```python
from build123d import *

# Parameters (mm, degrees)
F1_DEPTH  = 31.52012
F0_R      = 3.9989944529
F0_R_2    = 4.0304935081
F2_DEPTH  = 10.8295
F3_DEPTH  = 11.66704
F0_R_3    = 9.2896599899
F4_DEPTH  = 31.97776
F6_R      = 7.7262681343
F6_R_2    = 5.87306791
F7_DEPTH  = 7.37838
F9_DEPTH  = 23.31858
F0_R_4    = 5.7595758306
F0_R_5    = 5.6310949549
F10_DEPTH = 19.41152
F0_W      = 10.16
F0_H      = 21.1746012493
F11_DEPTH = 19.65592


# Not quite as in the source:
# - a feature names something its author has since deleted; it is built from what else it names
# - the program builds the solid bodies; features that only make, move or delete a surface that nothing else refers to are left out


with BuildPart() as f1:
    # F0 (on Front) → F1 (new body)
    with BuildSketch(Plane.XZ):
        with BuildLine():
            Line((-32.945703147, 0), (-53.0377118984, 0))
            Line((-53.0377118984, 0), (-53.0377118984, -13.8332377828))
            Line((-53.0377118984, -13.8332377828), (-5.08, -13.8332377828))
            Line((-5.08, -13.8332377828), (5.08, -13.8332377828))
            Line((5.08, -13.8332377828), (53.0377118984, -13.8332377828))
            Line((53.0377118984, -13.8332377828), (53.0377118984, 0))
            Line((53.0377118984, 0), (32.945703147, 0))
            add(Edge.make_bspline(
                [(32.945703147, 0), (28.5647447129, 0.0625927983), (19.8735598839, 0.1867678132), (20.1720018391, 8.6992646442), (20.3200084018, 12.9208741543)],
                knots=[0, 0, 0, 0, 0.5040691828, 1, 1, 1, 1], degree=3))
            ThreePointArc((20.3200084018, 12.9208741543), (23.9781287511, 23.6330514006), (20.3200084018, 34.345228647))
            Line((20.3200084018, 34.345228647), (20.3200084018, 57.3156722881))
            Line((20.3200084018, 57.3156722881), (-18.3321793468, 57.3156722881))
            Line((-18.3321793468, 57.3156722881), (-18.3321793468, 34.345228647))
            ThreePointArc((-18.3321793468, 34.345228647), (-21.9102829622, 23.6330514006), (-18.3321793468, 12.9208741543))
            add(Edge.make_bspline(
                [(-32.945703147, 0), (-28.5122837396, 0.0592468916), (-19.728591274, 0.176629532), (-18.7947032642, 8.6996856696), (-18.3321793468, 12.9208741543)],
                knots=[0, 0, 0, 0, 0.5047329952, 1, 1, 1, 1], degree=3))
        make_face()
        with BuildLine():
            ThreePointArc((6.2648822412, 33.191720318), (12.6390408842, 27.6514544893), (15.0142637131, 19.5469643528))
            ThreePointArc((15.0142637131, 19.5469643528), (-7.6843579979, 6.6481753784), (-7.1484956716, 32.75026411))
            ThreePointArc((-7.1484956716, 32.75026411), (-0.4938765731, 34.5531031225), (6.2648822412, 33.191720318))
        make_face(mode=Mode.SUBTRACT)
    extrude(amount=F1_DEPTH)

    # F0 (on Front) → F2 (join)
    with BuildSketch(Plane.XZ):
        with BuildLine():
            Line((-18.3321793468, 62.8374100943), (-18.3321793468, 57.3156722881))
            Line((-18.3321793468, 57.3156722881), (20.3200084018, 57.3156722881))
            Line((20.3200084018, 57.3156722881), (20.3200084018, 62.8374100943))
            add(Edge.make_bspline(
                [(20.3200084018, 62.8374100943), (20.1052749574, 65.5197235908), (19.6543576651, 71.15229537), (13.2786405866, 71.4934853371), (9.9391337225, 71.6721956254)],
                knots=[0, 0, 0, 0, 0.4762147029, 1, 1, 1, 1], degree=3))
            Line((9.9391337225, 71.6721956254), (-5.7426103852, 71.6721956254))
            add(Edge.make_bspline(
                [(-18.3321793468, 62.8374100943), (-18.0134703448, 65.7269619482), (-17.326155356, 71.9584530192), (-9.7862501304, 71.772123737), (-5.7426103852, 71.6721956254)],
                knots=[0, 0, 0, 0, 0.4637015156, 1, 1, 1, 1], degree=3))
        make_face()
        with Locations((-10.6017430574, 65.7269619482)):
            Circle(F0_R, mode=Mode.SUBTRACT)
        with Locations((13.0313078181, 65.7087189627)):
            Circle(F0_R_2, mode=Mode.SUBTRACT)
    extrude(amount=F2_DEPTH)

    # F0 (on Front) → F3 (join)
    with BuildSketch(Plane.XZ):
        with BuildLine():
            Line((-18.3321793468, 34.345228647), (-53.0377118984, 0))
            Line((-53.0377118984, 0), (-32.945703147, 0))
            add(Edge.make_bspline(
                [(-32.945703147, 0), (-28.5122837396, 0.0592468916), (-19.728591274, 0.176629532), (-18.7947032642, 8.6996856696), (-18.3321793468, 12.9208741543)],
                knots=[0, 0, 0, 0, 0.5047329952, 1, 1, 1, 1], degree=3))
            ThreePointArc((-18.3321793468, 12.9208741543), (-21.9102829622, 23.6330514006), (-18.3321793468, 34.345228647))
        make_face()
        with BuildLine():
            Line((53.0377118984, 0), (20.3200084018, 34.345228647))
            ThreePointArc((20.3200084018, 34.345228647), (23.9781287511, 23.6330514006), (20.3200084018, 12.9208741543))
            add(Edge.make_bspline(
                [(32.945703147, 0), (28.5647447129, 0.0625927983), (19.8735598839, 0.1867678132), (20.1720018391, 8.6992646442), (20.3200084018, 12.9208741543)],
                knots=[0, 0, 0, 0, 0.5040691828, 1, 1, 1, 1], degree=3))
            Line((32.945703147, 0), (53.0377118984, 0))
        make_face()
    extrude(amount=F3_DEPTH)

    # F0 (on Front) → F4 (join)
    with BuildSketch(Plane.XZ):
        with BuildLine():
            ThreePointArc((-7.1484956716, 32.75026411), (-7.6843579979, 6.6481753784), (15.0142637131, 19.5469643528))
            ThreePointArc((15.0142637131, 19.5469643528), (12.6390408842, 27.6514544893), (6.2648822412, 33.191720318))
            ThreePointArc((6.2648822412, 33.191720318), (-0.4938765731, 34.5531031225), (-7.1484956716, 32.75026411))
        make_face()
        with Locations((0, 19.5469643528)):
            Circle(F0_R_3, mode=Mode.SUBTRACT)
    extrude(amount=F4_DEPTH)

    # F6 (on offset) → F7 (cut)
    with BuildSketch(Plane.XY.offset(50.8)):
        with Locations((0, -19.8897793889)):
            Circle(F6_R)
        with Locations((0, -19.8897793889)):
            Circle(F6_R_2, mode=Mode.SUBTRACT)
    extrude(amount=F7_DEPTH, mode=Mode.SUBTRACT)

    # F9 (cut): a face of the model
    f9_faces = [f1.faces().sort_by_distance(p)[0] for p in [
        (0, -19.8897793889, 57.3156722881),
    ]]
    extrude(f9_faces, amount=-F9_DEPTH, mode=Mode.SUBTRACT)

    # F0 (on Front) → F10 (join)
    with BuildSketch(Plane.XZ):
        with BuildLine():
            Line((-5.08, -13.8332377828), (-53.0377118984, -13.8332377828))
            Line((-53.0377118984, -13.8332377828), (-53.0377118984, -21.0930503504))
            add(Edge.make_bspline(
                [(-53.0377118984, -21.0930503504), (-53.4005944702, -25.2780429079), (-54.7251608325, -36.2581171884), (-35.7792689312, -35.346119388), (-25.8417483085, -35.0078390322)],
                knots=[0, 0, 0, 0, 0.3981682681, 1, 1, 1, 1], degree=3))
            Line((-25.8417483085, -35.0078390322), (-5.08, -35.0078390322))
            Line((-5.08, -35.0078390322), (-5.08, -13.8332377828))
        make_face()
        with Locations((-45.0574053683, -26.3939229293)):
            Circle(F0_R_4, mode=Mode.SUBTRACT)
        with BuildLine():
            Line((53.0377118984, -13.8332377828), (5.08, -13.8332377828))
            Line((5.08, -13.8332377828), (5.08, -35.0078390322))
            Line((5.08, -35.0078390322), (35.7808830812, -35.0078390322))
            add(Edge.make_bspline(
                [(53.0377118984, -21.0930503504), (52.1158724207, -25.6188280404), (49.8115979989, -34.1905224475), (41.3452471932, -34.893061815), (35.7808830812, -35.0078390322)],
                knots=[0, 0, 0, 0, 0.4907243677, 1, 1, 1, 1], degree=3))
            Line((53.0377118984, -21.0930503504), (53.0377118984, -13.8332377828))
        make_face()
        with Locations((43.7321887989, -26.8356617858)):
            Circle(F0_R_5, mode=Mode.SUBTRACT)
    extrude(amount=F10_DEPTH)

    # F0 (on Front) → F11 (join)
    with BuildSketch(Plane.XZ):
        with Locations((0, -24.4205384075)):
            Rectangle(F0_W, F0_H)
    extrude(amount=F11_DEPTH)


solid = f1.part
```
CAD build for the part. Positions are in the model's coordinates, mm. A direction names the side the tool comes from. Round coordinates to 2 decimals unless told otherwise and drop trailing zeros. Write each loop counter-clockwise with the first axis right and the second up, starting at its lowest first coordinate (ties: lowest second). Pieces come first, ordered by that corner, then holes.
Item 1: Band-saw the part on A-A on x = 0. Write the cut outline in (y, z), then the cut area to 3 significant figures.
Filled in:
outline: (-31.98, 4.53) - (-31.52, 4.53) - (-31.52, -13.83) - (-19.66, -13.83) - (-19.66, -35.01) - (0, -35.01) - (0, 10.26) - (-31.98, 10.26) - close; (-31.98, 28.84) - (0, 28.84) - (0, 71.67) - (-10.83, 71.67) - (-10.83, 57.32) - (-12.16, 57.32) - (-12.16, 50.8) - (-14.02, 50.8) - (-14.02, 34) - (-25.76, 34) - (-25.76, 50.8) - (-27.62, 50.8) - (-27.62, 57.32) - (-31.52, 57.32) - (-31.52, 34.56) - (-31.98, 34.56) - close
area: 1,940 mm2
Item 2: Mould opens along X. For faces 1 (the flat face through (20.32, -16, 45)), 2 (the flat face through (1, -10.83, 65)), 3 (the cylindrical face through (-0.765, -25.713, 42.516)) say: released by +X, released by -X, zero draft, split by the parting line, or undercut.
Filled in:
face 1: released by +X
face 2: zero draft
face 3: undercut
Item 3: Drill centre lines: L1, parallel to Z at x = 0, y = -21; L2, parallel to X at y = -2, z = 63.5; L3, parallel to Y at x = 24.5, z = -2.5. Where is each one in solid material? Low to high.
Filled in:
L1: z = -13.83 to 10.26, 28.84 to 34
L2: x = -18.26 to -13.92, -7.28 to 9.66, 16.4 to 20.27
L3: y = -31.52 to 0
Item 4: Band-saw the part on B-B on z = -10.5. Write the cut outline in (x, y).
Filled in:
outline: (-53.04, -31.52) - (53.04, -31.52) - (53.04, 0) - (-53.04, 0) - close
Item 5: Drop flat-ended pins along their axis: pin 1 Ø1 at (y, z) = (-5, 18) entering from -X; pin 2 Ø4 at (x, y) = (2, -23) entering from +Z; pin 3 Ø5 at (y, z) = (-25.5, 58) entering from -X; pin 4 Ø10 at (x, z) = (-23.5, 38.5) entering from -Y. Give the stop position or say it passes through.
Filled in:
pin 1: stops at x = -35.35
pin 2: stops at z = 34
pin 3: stops at x = -18.33
pin 4: passes through
Item 6: Band-saw the part on C-C on y = -5.5. Give the number of separate pieces and of enclosed holes in the cut face, then the cut area to 3 significant figures.
Filled in:
separate pieces: 1
enclosed holes: 5
area: 6,990 mm2
Item 7: Tool access for faces 4 (the flat face through (-30, -19.412, -25)), 5 (the flat face through (2, -14, 50.8)), 6 (the flat face through (6.5, -31.978, 26.4)), 7 (the flat face through (5, -10, -35.008)), 8 (the flat face through (43, -21, 0)): list every direction of +Z, -Z, +X, -X, +Y, -Y with a clear straight run to the whole face (end or side of a thin tool).
Filled in:
face 4: -Z, -X, -Y
face 5: +Z
face 6: +Z, -Z, +X, -X, -Y
face 7: -Z, +X, +Y, -Y
face 8: +Z, +X, -Y
